from build123d import *

# Parameters (mm, degrees)
SKETCH1_R               = 25.4
BOSS_EXTRUDE1_DEPTH     = 7.62
SKETCH2_W               = 33.02
SKETCH2_H               = 25.4
BOSS_EXTRUDE2_DEPTH     = 25.4
SKETCH4_R               = 6.35
CUT_EXTRUDE1_DEPTH      = 9.89
CUT_EXTRUDE1_DEPTH_BACK = 42.91
SCALE1_SCALE            = 3
FILLET1_R               = 10.16


with BuildPart() as part:
    # Sketch1 → Boss-Extrude1 (new body)
    with BuildSketch(Plane(origin=(0, 0, 0), x_dir=(1, 0, 0), z_dir=(0, 1, 0))):
        Circle(SKETCH1_R)
    extrude(amount=BOSS_EXTRUDE1_DEPTH)

    # Sketch2 → Boss-Extrude2 (add)
    with BuildSketch(Plane(origin=(0, 7.62, 0), x_dir=(1, 0, 0), z_dir=(0, 1, 0))):
        Rectangle(SKETCH2_W, SKETCH2_H)
    extrude(amount=BOSS_EXTRUDE2_DEPTH)

    # Sketch4 → Cut-Extrude1 (cut, two sides)
    with BuildSketch(Plane.ZY.offset(16.51)) as cut_extrude1_sk:
        with Locations((0, 20.32)):
            Circle(SKETCH4_R)
    extrude(amount=CUT_EXTRUDE1_DEPTH, mode=Mode.SUBTRACT)
    extrude(cut_extrude1_sk.sketch, amount=-CUT_EXTRUDE1_DEPTH_BACK, mode=Mode.SUBTRACT)


with BuildPart() as part_1:
    # Scale1: scaled about (0, 12.489824254, 0)
    add(part.part.scale(SCALE1_SCALE).moved(Location((0, -24.979648508, 0))))

    # Fillet1
    fillet1_edges = [part_1.edges().sort_by_distance(p)[0] for p in [
        (0, 74.080351492, 38.1),
        (49.53, -2.119648508, 0),
        (49.53, 35.980351492, 38.1),
        (0, -2.119648508, -38.1),
        (49.53, 35.980351492, -38.1),
        (-49.53, -2.119648508, 0),
        (-49.53, 35.980351492, -38.1),
        (0, -2.119648508, 38.1),
        (-49.53, 35.980351492, 38.1),
        (49.53, 74.080351492, 0),
        (0, 74.080351492, -38.1),
        (-49.53, 74.080351492, 0),
    ]]
    fillet(fillet1_edges, radius=FILLET1_R)


solid = part_1.part
Model file for the job. Use its own axes, mm. A direction names the side the tool comes from. Give positions to 0.01 mm unless a question says otherwise; leave off trailing zeros. Order: outer loops, then holes, each group sorted by start corner. A loop starts at its lowest first (then second) coordinate and runs counter-clockwise, first axis right, second up. Notation, with made-up numbers: M 57.5,-24.75 L 91.5,-24.75 A21 cw 91.5,-9.75 Z; hole C 18,42.5 d6. An arc over 180 degrees is marked long. Put each result on its own line as item: value. Start each with the question number.
(1) Band-saw the part on D-D on y = 0.5. Give the cut face in (x, z), then the cut area to 3 significant figures.
(2) Pin check, flat tips, straight feed: pin 1 Ø17 at (y, z) = (48, -9) entering from +X; pin 2 Ø5 at (x, z) = (53, 56.5) entering from +Y; pin 3 Ø5 at (x, y) = (10.5, -9.5) entering from -Z. Stop position of each tip, or through.
(3) Band-saw the part on A-A on z = 0. Give the cut face in (x, y), then the cut area to 3 significant figures.
(4) Band-saw the part on C-C on x = 6.5. Give the cut face in (y, z).
(5) Band-saw the part on B-B on y = 27. Give the cut face in (x, z), then the cut area to 3 significant figures.
(6) Tool access for faces 1 (the face through (-1, 36, 38.1)), 2 (the face through (49.53, 17, -6)), 3 (the face through (46.633, 36.372, -35.045)): list every direction of +Z, -Z, +X, -X, +Y, -Y with a clear straight run to the whole face (end or side of a thin tool).
(7) Drill centre lines: L1, parallel to Y at x = -17, z = 0; L2, parallel to Y at x = -40, z = -51; L3, parallel to Y at x = -13, z = 8.5. Where is each one in solid material? Low to high. Write a range as [from, to].
Results below:
1. outline: M -52.88,-27.94 A13.51 ccw -39.37,-41.45 L 39.37,-41.45 A13.51 ccw 52.88,-27.94 L 52.88,27.94 A13.51 ccw 39.37,41.45 L -39.37,41.45 A13.51 ccw -52.88,27.94 Z
1. area: 8,610 mm2
2. pin 1: stops at x = 49.53
2. pin 2: stops at y = -2.12
2. pin 3: stops at z = -75.78
3. outline: M -76.2,-24.98 L 76.2,-24.98 L 76.2,-2.12 L 59.69,-2.12 A10.16 cw 49.53,8.04 L 49.53,16.93 L -49.53,16.93 L -49.53,8.04 A10.16 cw -59.69,-2.12 L -76.2,-2.12 Z; M -49.53,55.03 L 49.53,55.03 L 49.53,63.92 A10.16 ccw 39.37,74.08 L -39.37,74.08 A10.16 ccw -49.53,63.92 Z
3. area: 7,260 mm2
4. outline: M -24.98,-75.92 L -2.12,-75.92 L -2.12,-48.26 A10.16 cw 8.04,-38.1 L 63.92,-38.1 A10.16 ccw 74.08,-27.94 L 74.08,27.94 A10.16 ccw 63.92,38.1 L 8.04,38.1 A10.16 cw -2.12,48.26 L -2.12,75.92 L -24.98,75.92 Z; hole C 35.98,0 d38.1
5. outline: M -49.53,-27.94 A10.16 ccw -39.37,-38.1 L 39.37,-38.1 A10.16 ccw 49.53,-27.94 L 49.53,-16.8 L -49.53,-16.8 Z; M -49.53,16.8 L 49.53,16.8 L 49.53,27.94 A10.16 ccw 39.37,38.1 L -39.37,38.1 A10.16 ccw -49.53,27.94 Z
5. area: 4,130 mm2
6. face 1: +Z, +X, -X, +Y
6. face 2: +Z, -Z, +X, +Y
6. face 3: -Z, +X, +Y
7. L1: y = [-24.98, 16.93], [55.03, 74.08]
7. L2: y = [-24.98, -2.12]
7. L3: y = [-24.98, 18.93], [53.03, 74.08]
